Answer from the drawing. Dimensions are ordinates in mm from the lowest x, y and z of the part. A direction names the side the tool comes from. Round coordinates to 2 decimals unless told otherwise and drop trailing zeros. Loops run counter-clockwise (first coordinate to the right, second up) from the corner with the lowest first, then second, coordinate; pieces in that order, holes last. Notation, with made-up numbers: (59, 64) - (100, 64) arc R29 cw to (100, 89) - close; hole circle Ø5 at (-36, -12). An arc over 180 degrees is marked (long way). Answer as CSV lines item,"result". Start each with the question number.
Q1. For the marked faces 1, 2, 3, 4 and 5, determine the directions among +Z, -Z, +X, -X, +Y, -Y from which every point of the face is accessible in a straight line to the end or side of a thin tool.
Q2. Section D-D on z = 28.25 is taken. Count the separate pieces of the cut face and the enclosed holes in it.
Q3. Straight lines are drawn through the part: L1, parallel to Y at x = 57.5, z = 21; L2, parallel to X at y = 18.5, z = 22.5 (1 decimal); L3, parallel to Z at x = 44, y = 6.5. For each, find the intervals that lie inside material, in ascending order. Write a range as [from, to].
Q4. Section A-A on y = 18.5 is taken. Write down the section's boundary in (x, z) (1 decimal), then the cut area to 3 significant figures.
Q5. The mould has two halves that part along Z. Classify the marked faces 6, 7, 8 and 9: +Z half, -Z half, draft (parallel to the pull), parting line (faces both ways), or undercut.
Q6. Each of these flat-tipped pins is pushed along its axis until it touches: pin 1 Ø5 at (x, z) = (16, 24) entering from +Y; pin 2 Ø3 at (y, z) = (8, 20.5) entering from -X; pin 3 Ø9.5 at (x, y) = (35.69, 9.93) entering from +Z; pin 4 Ø8 at (x, y) = (34.5, 4) entering from -Z. Where does it stop, or does it pass through?
Q7. Section C-C on z = 17.25 is taken. Write down the section's boundary in (x, y).
Q8. Section B-B on x = 23.5 is taken. Write down the section's boundary in (y, z).
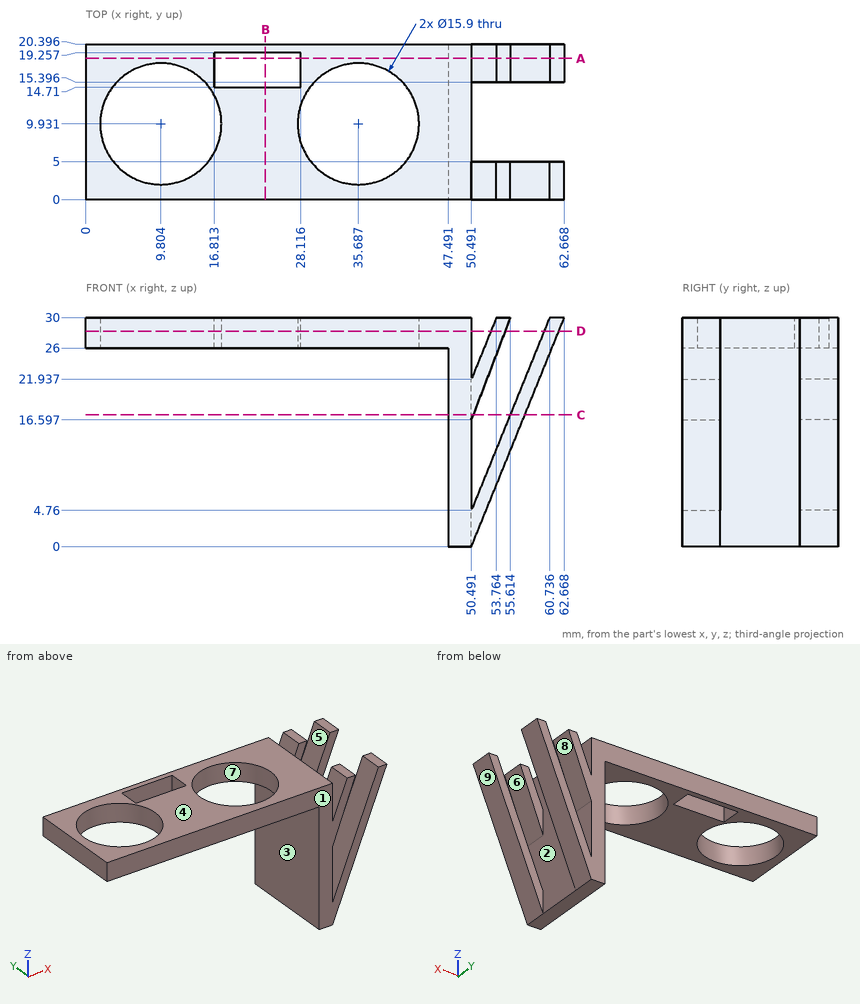
Findings:
1,face 1,"+Z, -Z, +X, -X, -Y"
1,face 2,"none"
1,face 3,"-Z, -X, +Y, -Y"
1,face 4,"+Z, +X, -X, +Y, -Y"
1,face 5,"+Y, -Y"
2,separate pieces,"5"
2,enclosed holes,"3"
3,L1,"y = [0, 5], [15.4, 20.4]"
3,L2,"x = [47.5, 50.5], [50.7, 52.7], [57.7, 59.6]"
3,L3,"z = [26, 30]"
4,outline,"(0, 26) - (16.8, 26) - (16.8, 30) - (0, 30) - close; (28.1, 26) - (47.5, 26) - (47.5, 0) - (50.5, 0) - (62.7, 30) - (60.7, 30) - (50.5, 4.8) - (50.5, 16.6) - (55.6, 30) - (53.8, 30) - (50.5, 21.9) - (50.5, 30) - (28.1, 30) - close"
4,area,"309 mm^2"
5,face 6,"undercut"
5,face 7,"draft"
5,face 8,"undercut"
5,face 9,"-Z half"
6,pin 1,"stops at y = 20.4"
6,pin 2,"stops at x = 47.49"
6,pin 3,"passes through"
6,pin 4,"stops at z = 26"
7,outline,"(47.49, 0) - (50.74, 0) - (50.74, 5) - (50.49, 5) - (50.49, 15.4) - (50.74, 15.4) - (50.74, 20.4) - (47.49, 20.4) - close; (55.56, 0) - (57.49, 0) - (57.49, 5) - (55.56, 5) - close; (55.56, 15.4) - (57.49, 15.4) - (57.49, 20.4) - (55.56, 20.4) - close"
8,outline,"(0, 26) - (14.71, 26) - (14.71, 30) - (0, 30) - close; (19.26, 26) - (20.4, 26) - (20.4, 30) - (19.26, 30) - close"
